Input: part model. Units: mm. Frame: model coordinates. Round coordinates to 2 decimals unless told otherwise and drop trailing zeros. Loops run counter-clockwise (first coordinate to the right, second up) from the corner with the lowest first, then second, coordinate; pieces in that order, holes last. Notation, with made-up numbers: (-7.75, 24.5) -> (37.25, 24.5) arc R16 cw to (37.25, 29.5) -> close; hole circle Ø8 at (-26, 3). An arc over 180 degrees is marked (long way). Answer in a Markdown table with one row per item. Add a question column.
Q1. Section B-B, the plane z = 0.3. Output: boundary loops of the cut face in (x, y), and give its area (3 significant figures).
Q2. Pin query (flat end, axial travel): pin 1 (0.8 mm diameter, centred on x = -0.5, y = 5.5, fed in from +Z); pin 2 (0.8 mm diameter, centred on x = -0.5, y = 9, fed in from -Z). Return the tip coordinate at first contact, or that it passes through.
Q3. Section A-A, the plane y = 6.5. Output: boundary loops of the cut face in (x, z).
Q4. Ray query, L1, parallel to X at y = 3.75, z = 1.55. Return the intervals inside material, ascending. Write a range as from..to.
Autodesk Inventor part; units mm, degrees
ref_plane "YZ Plane" through (0, 0, 0) normal (1, 0, 0) x (0, 1, 0)
ref_plane "XZ Plane" through (0, 0, 0) normal (0, 1, 0) x (-1, 0, 0)
ref_plane "XY Plane" through (0, 0, 0) normal (0, 0, 1) x (1, 0, 0)
sketch "Sketch1" plane through (0, 0, 0) normal (0, 0, 1) x (1, 0, 0)
  line L0 (0, 0) -> (42, 0)
  line L1 (42, 0) -> (42, 14)
  line L2 (42, 14) -> (0, 14)
  line L3 (0, 14) -> (0, 0)
  dimension "d0" = 42
  dimension "d1" = 14
extrude "Extrusion1" add sketch "Sketch1" along normal blind 2
sketch "Sketch2" plane through (42, 0, 0) normal (1, 0, 0) x (0, 0, -1)
  line L0 (0, 14) -> (-2, 14)
  line L1 (-2, 0) -> (-2, 14)
  line L2 (0, 0) -> (-2, 0)
  line L3 (-1.15, 0) -> (-0.85, 0)
  line L4 (-0.85, 0) -> (-0.85, 14)
  line L5 (-0.85, 14) -> (-1.15, 14)
  line L6 (-1.15, 14) -> (-1.15, 0)
  dimension "d4" = 0.85
  dimension "d5" = 0.3
extrude "Extrusion2" add sketch "Sketch2" along normal blind 1 contours L4 L2 L6 L0
sketch "Sketch3" plane through (0, 0, 0) normal (-1, 0, 0) x (0, 0, 1)
  line L0 (0.85, 14) -> (1.15, 14)
  line L1 (1.15, 14) -> (1.15, 0)
  line L2 (0.85, 14) -> (1.15, 14)
  line L3 (1.15, 14) -> (1.15, 0)
  line L4 (1.15, 0) -> (0.85, 0)
  line L5 (0.85, 0) -> (0.85, 14)
extrude "Extrusion3" add sketch "Sketch3" along normal blind 1
properties part number "Voorplaat"
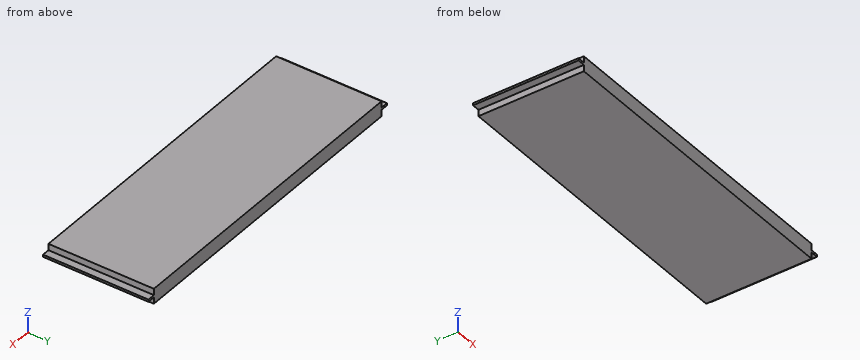
Answer block:
| question | item | result |
|---|---|---|
| 1 | outline | (0, 0) -> (42, 0) -> (42, 14) -> (0, 14) -> close |
| 1 | area | 588 mm^2 |
| 2 | pin 1 | z = 1.15 |
| 2 | pin 2 | z = 0.85 |
| 3 | outline | (-1, 0.85) -> (0, 0.85) -> (0, 0) -> (42, 0) -> (42, 0.85) -> (43, 0.85) -> (43, 1.15) -> (42, 1.15) -> (42, 2) -> (0, 2) -> (0, 1.15) -> (-1, 1.15) -> close |
| 4 | L1 | 0..42 |
